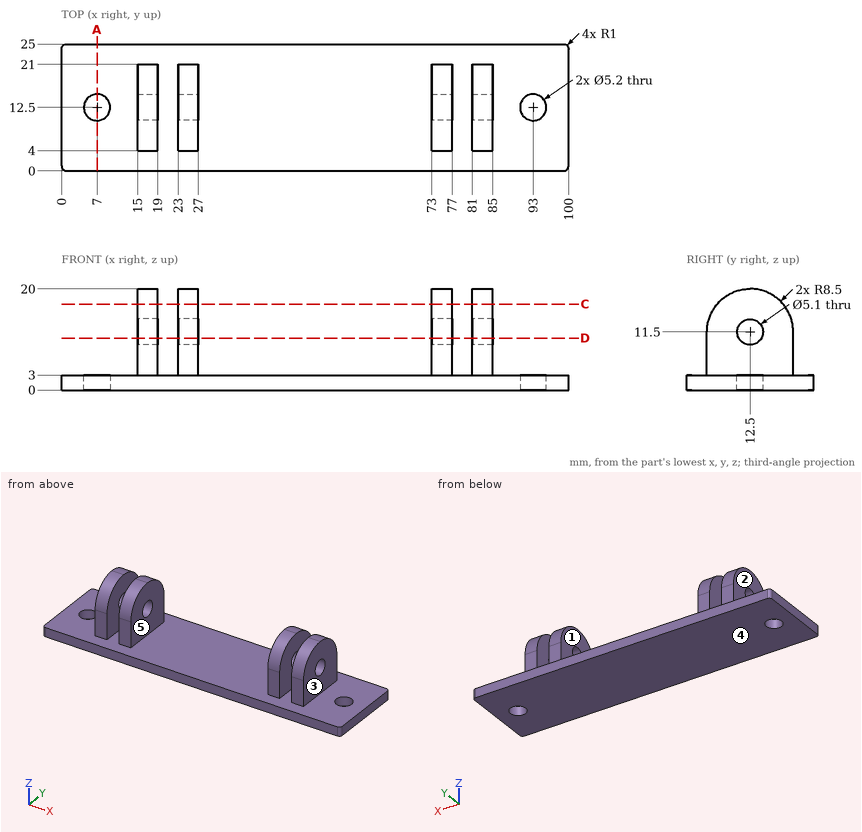
Drawing for the job (mm, zero at the part's lowest x, y, z). A direction names the side the tool comes from. Round coordinates to 2 decimals unless told otherwise and drop trailing zeros. Order: outer loops, then holes, each group sorted by start corner. A loop starts at its lowest first (then second) coordinate and runs counter-clockwise, first axis right, second up. Notation, with made-up numbers: M -25.5,70.25 L 8.5,70.25 A23 ccw 8.5,108.25 Z; hole C 39.25,-26.5 d9. An arc over 180 degrees is marked long. Use one line per item in the form item = value.
Q1. Probe L1, parallel to X at y = 12.5, z = 17.5; L2, parallel to Z at x = 82.25, y = 12.5; L3, parallel to Y at x = 93, z = 0.7. List the from-to ranges inside material, lowest first.
Recorded:
L1 = 15 to 19, 23 to 27, 73 to 77, 81 to 85
L2 = 0 to 8.95, 14.05 to 20
L3 = 0 to 9.9, 15.1 to 25
Q2. Saw through at C-C on z = 17. Give the cut face in (x, y).
Recorded:
outline = M 15,6.02 L 19,6.02 L 19,18.98 L 15,18.98 Z; M 23,6.02 L 27,6.02 L 27,18.98 L 23,18.98 Z; M 73,6.02 L 77,6.02 L 77,18.98 L 73,18.98 Z; M 81,6.02 L 85,6.02 L 85,18.98 L 81,18.98 Z
Q3. Flat gauge pins, fed straight in: P1, Ø3, axis at x = 83, z = 6, coming from the +Y side; P2, Ø4, axis at x = 48.5, y = 10, coming from the +Z side; P3, Ø3, axis at y = 12.5, z = 11.5, coming from the -X side; P4, Ø8, axis at y = 19, z = 13.5, coming from the +X side. Where does each tip first touch, or does it go through?
Recorded:
P1 = 21
P2 = 3
P3 = through
P4 = 85
Q4. Saw through at A-A on x = 7. Give the cut face in (y, z).
Recorded:
outline = M 0,0 L 9.9,0 L 9.9,3 L 0,3 Z; M 15.1,0 L 25,0 L 25,3 L 15.1,3 Z
Q5. Two-plate mould, pull along X, no slides. Class the marked faces 1, 2 and 3: +X half, -X half, draft (parallel to the pull), parting line (faces both ways), or undercut.
Recorded:
face_1 = undercut
face_2 = -X half
face_3 = +X half
Q6. Saw through at D-D on z = 10.25. State how many separate pieces and enclosed holes the cut face has, then the cut area to 3 significant figures.
Recorded:
separate_pieces = 8
enclosed_holes = 0
area = 201 mm^2
Q7. Which spindle directions (+Z, -Z, +X, -X, +Y, -Y) get a long thin tool onto all of the face, cutting with end or side? Do the marked faces 4 and 5. Say none if no direction does.
Recorded:
face_4 = -Z, +X, -X, +Y, -Y
face_5 = +Z, +Y, -Y
